from build123d import *

# Parameters (mm, degrees)
SKETCH2_R           = 2.65
BOSS_EXTRUDE4_DEPTH = 6
CUT_EXTRUDE2_DEPTH  = 88.793483499


with BuildPart() as part:
    # Sketch2 → Boss-Extrude4 (new body)
    with BuildSketch(Plane.XY):
        with BuildLine():
            add(Edge.make_bspline(
                [(67.5, 17.578928476), (65.61016752, 17.502615465), (60.634413429, 17.271238409), (53.13057404, 16.789010877), (47.524682176, 16.292383273), (45, 16.035396523)],
                knots=[0.381536428, 0.381536428, 0.381536428, 0.381536428, 0.390812303, 0.405965006, 0.418410632, 0.418410632, 0.418410632, 0.418410632], degree=3))
            ThreePointArc((45, 16.035396523), (62.750493933, 0), (45, -16.035396523))
            add(Edge.make_bspline(
                [(45, -16.035396523), (47.524682176, -16.292383273), (53.13057404, -16.789010877), (60.634413429, -17.271238409), (65.61016752, -17.502615465), (67.5, -17.578928476)],
                knots=[0.581589368, 0.581589368, 0.581589368, 0.581589368, 0.594034994, 0.609187697, 0.618463572, 0.618463572, 0.618463572, 0.618463572], degree=3))
            ThreePointArc((67.5, -17.578928476), (85.803106629, 0), (67.5, 17.578928476))
        make_face()
        with Locations((68.209851787, 0)):
            Circle(SKETCH2_R, mode=Mode.SUBTRACT)
    extrude(amount=BOSS_EXTRUDE4_DEPTH)

    # Sketch4 → Cut-Extrude2 (cut, through all)
    with BuildSketch(Plane.XY.offset(6)):
        with BuildLine():
            Line((65.5273107, 17.495020066), (67.512104385, 17.279172769))
            ThreePointArc((67.512104385, 17.279172769), (85.503106629, 0), (67.512104385, -17.279172769))
            Line((67.512104385, -17.279172769), (65.5273107, -17.495020066))
            add(Edge.make_bspline(
                [(65.5273107, -17.495020066), (66.184811673, -17.524419912), (66.842377464, -17.55237313), (67.5, -17.578928476)],
                knots=[0.615235759, 0.615235759, 0.615235759, 0.615235759, 0.618463572, 0.618463572, 0.618463572, 0.618463572], degree=3))
            ThreePointArc((67.5, -17.578928476), (85.803106629, 0), (67.5, 17.578928476))
            add(Edge.make_bspline(
                [(67.5, 17.578928476), (66.842377464, 17.55237313), (66.184811673, 17.524419912), (65.5273107, 17.495020066)],
                knots=[0.381536428, 0.381536428, 0.381536428, 0.381536428, 0.384764241, 0.384764241, 0.384764241, 0.384764241], degree=3))
        make_face()
        with BuildLine():
            ThreePointArc((48.197537186, -16.3434678), (63.050493933, 0), (48.197537186, 16.3434678))
            add(Edge.make_bspline(
                [(48.197537186, 16.3434678), (47.131160592, 16.246385916), (46.065284113, 16.143831519), (45, 16.035396523)],
                knots=[0.413159228, 0.413159228, 0.413159228, 0.413159228, 0.418410632, 0.418410632, 0.418410632, 0.418410632], degree=3))
            ThreePointArc((45, 16.035396523), (62.750493933, 0), (45, -16.035396523))
            add(Edge.make_bspline(
                [(45, -16.035396523), (46.065284113, -16.143831519), (47.131160592, -16.246385916), (48.197537186, -16.3434678)],
                knots=[0.581589368, 0.581589368, 0.581589368, 0.581589368, 0.586840772, 0.586840772, 0.586840772, 0.586840772], degree=3))
        make_face()
    extrude(amount=-CUT_EXTRUDE2_DEPTH, mode=Mode.SUBTRACT)


solid = part.part
Read the model definition and answer for the solid it produces. Units are mm, in the model's axes. Round coordinates to 2 decimals unless told otherwise and drop trailing zeros. Write each loop counter-clockwise with the first axis right and the second up, starting at its lowest first coordinate (ties: lowest second). Pieces come first, ordered by that corner, then holes. Notation, with made-up numbers: (48, -17.5) - (64, -17.5) arc R6 cw to (64, -11.5) - close; hole circle Ø2 at (76, 36.5). An arc over 180 degrees is marked (long way). Use a Markdown table: item, result.
(1) Straight lines are drawn through the part: line 1 along Y through (x, z) = (54, 2.5); line 2 along Y through (x, z) = (69, 4.5); line 3 along Y through (x, z) = (83, 0.5). For each, find the intervals that lie inside material, in ascending order. Write a range as [from, to].
Reported:
| item | result |
|---|---|
| line 1 | [-16.82, -14.67], [14.67, 16.82] |
| line 2 | [-17.28, -2.53], [2.53, 17.28] |
| line 3 | [-8.96, 8.96] |
(2) The mould has two halves that part along X. Classify faces 1 (the cylindrical face through (70.737, 0.796, 2.958)), 2 (the flat face through (66.51, 17.39, 3.04)), 3 (the cylindrical face through (63.047, -0.339, 3.042)): released by +X, released by -X, zero draft, split by the parting line, or undercut.
Reported:
| item | result |
|---|---|
| face 1 | undercut |
| face 2 | released by +X |
| face 3 | released by -X |
(3) The part is cut by section D-D (y = 8.5). Write down the section's boundary in (x, z), then the cut area to 3 significant figures.
Reported:
| item | result |
|---|---|
| outline | (60.68, 0) - (83.27, 0) - (83.27, 6) - (60.68, 6) - close |
| area | 136 mm2 |
(4) The part is cut by section B-B (x = 68.5). Write down the section's boundary in (y, z), then the cut area to 3 significant figures.
Reported:
| item | result |
|---|---|
| outline | (-17.29, 0) - (-2.63, 0) - (-2.63, 6) - (-17.29, 6) - close; (2.63, 0) - (17.29, 0) - (17.29, 6) - (2.63, 6) - close |
| area | 176 mm2 |
(5) The part is cut by section C-C (x = 80). Write down the section's boundary in (y, z).
Reported:
| item | result |
|---|---|
| outline | (-12.65, 0) - (12.65, 0) - (12.65, 6) - (-12.65, 6) - close |
(6) The part is cut by section A-A (y = 0). Write down the section's boundary in (x, z), then the cut area to 3 significant figures.
Reported:
| item | result |
|---|---|
| outline | (63.05, 0) - (65.56, 0) - (65.56, 6) - (63.05, 6) - close; (70.86, 0) - (85.5, 0) - (85.5, 6) - (70.86, 6) - close |
| area | 103 mm2 |
(7) Each of these flat-tipped pins is pushed along its axis until it touches: pin 1 Ø2 at (x, z) = (62.5, 4) entering from +Y; pin 2 Ø1.5 at (x, z) = (74, 1) entering from +Y; pin 3 Ø2 at (y, z) = (-7, 5) entering from -X. Where does it stop, or does it pass through?
Reported:
| item | result |
|---|---|
| pin 1 | y = 17.4 |
| pin 2 | y = 16.54 |
| pin 3 | x = 60.97 |
